from build123d import *

# Parameters (mm, degrees)
SKETCH1_W           = 50
SKETCH1_H           = 80
BOSS_EXTRUDE1_DEPTH = 6
BOSS_EXTRUDE2_DEPTH = 16
FILLET1_R           = 5
FILLET2_R           = 5
SKETCH3_R           = 2.6
CUT_EXTRUDE1_DEPTH  = 10
SKETCH4_W           = 24
SKETCH4_H           = 47.75
CUT_EXTRUDE3_DEPTH  = 20
SKETCH5_W           = 23.965270804
SKETCH5_H           = 10
BOSS_EXTRUDE3_DEPTH = 16
FILLET3_R           = 5


with BuildPart() as part:
    # Sketch1 → Boss-Extrude1 (new body)
    with BuildSketch(Plane(origin=(0, 0, 0), x_dir=(1, 0, 0), z_dir=(0, 1, 0))):
        with Locations((-55.945507312, -78.533333333)):
            Rectangle(SKETCH1_W, SKETCH1_H)
    extrude(amount=BOSS_EXTRUDE1_DEPTH)

    # Sketch2 → Boss-Extrude2 (add)
    with BuildSketch(Plane(origin=(0, 6, 0), x_dir=(1, 0, 0), z_dir=(0, 1, 0))):
        Polygon((-80.945507312, -38.533333333), (-80.945507312, -118.533333333), (-50.945507312, -118.533333333), (-50.945507312, -58.292829883), (-73.945507312, -58.292829883), align=None)
        Polygon((-35.945507312, -44.292829883), (-35.945507312, -118.533333333), (-30.945507312, -118.533333333), (-30.945507312, -38.533333333), (-56.945507312, -44.292829883), align=None)
    extrude(amount=BOSS_EXTRUDE2_DEPTH)

    # Fillet1
    fillet1_edges = [part.edges().sort_by_distance(p)[0] for p in [
        (-50.945507312, 14, 58.292829883),
        (-73.945507312, 14, 58.292829883),
    ]]
    fillet(fillet1_edges, radius=FILLET1_R)

    # Fillet2
    fillet2_edges = [part.edges().sort_by_distance(p)[0] for p in [
        (-35.945507312, 14, 44.292829883),
    ]]
    fillet(fillet2_edges, radius=FILLET2_R)

    # Sketch3 → Cut-Extrude1 (cut)
    with BuildSketch(Plane(origin=(0, 0, 58.292829883), x_dir=(-1, 0, 0), z_dir=(0, 0, -1))):
        with Locations((59.128917582, 16.867919386)):
            Circle(SKETCH3_R)
        with Locations((67.228917582, 16.867919386)):
            Circle(SKETCH3_R)
    extrude(amount=-CUT_EXTRUDE1_DEPTH, mode=Mode.SUBTRACT)

    # Sketch4 → Cut-Extrude3 (cut)
    with BuildSketch(Plane.XZ):
        with Locations((-65.945507312, 92.158333333)):
            Rectangle(SKETCH4_W, SKETCH4_H)
    extrude(amount=-CUT_EXTRUDE3_DEPTH, mode=Mode.SUBTRACT)

    # Sketch5 → Boss-Extrude3 (add)
    with BuildSketch(Plane.XY.offset(68.283333333)):
        with Locations((-65.928142714, 5)):
            Rectangle(SKETCH5_W, SKETCH5_H)
    extrude(amount=BOSS_EXTRUDE3_DEPTH)

    # Fillet3
    fillet3_edges = [part.edges().sort_by_distance(p)[0] for p in [
        (-50.945507312, 14, 118.533333333),
        (-30.945507312, 11, 118.533333333),
        (-80.945507312, 11, 118.533333333),
    ]]
    fillet(fillet3_edges, radius=FILLET3_R)


solid = part.part
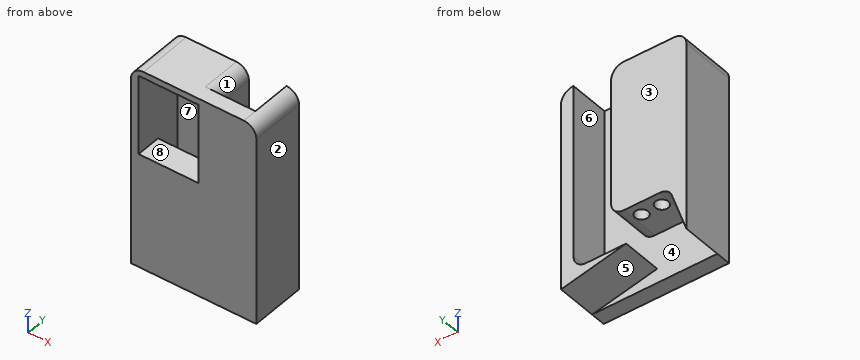
Part model, mm, in its own coordinate system. Face numbers are marked on the shaded views. A direction names the side the tool comes from. Coordinates: 2 decimals unless noted, no trailing zeros. Write each loop counter-clockwise with the first axis right and the second up, starting at its lowest first coordinate (ties: lowest second). Pieces come first, ordered by that corner, then holes. Notation, with made-up numbers: M 58.25,52 L 64.25,52 A24 ccw 64.25,66 Z; hole C 61.25,-34 d5. An arc over 180 degrees is marked long. Return JSON: item names as keys, results as strings.
1. Saw through at A-A, the plane y = 12. Write the cut outline in (x, z), then the cut area to 3 significant figures.
Determined:
{"outline": "M -80.95,38.53 L -75.13,54.96 A5 cw -70.41,58.29 L -55.95,58.29 A5 ccw -50.95,63.29 L -50.95,113.53 A5 ccw -55.95,118.53 L -75.95,118.53 A5 ccw -80.95,113.53 Z; M -56.95,44.29 L -30.95,38.53 L -30.95,113.53 A5 ccw -35.95,118.53 L -35.95,49.29 A5 cw -40.95,44.29 Z; hole M -77.95,68.28 L -53.95,68.28 L -53.95,116.03 L -77.95,116.03 Z", "area": "1,160 mm²"}
2. Flat gauge pins, fed straight in: pin 1 Ø5 at (x, z) = (-45, 89) entering from +Y; pin 2 Ø3 at (x, y) = (-59.5, 11.5) entering from -Z; pin 3 Ø4 at (x, y) = (-59.13, 16.87) entering from -Z. Where does each tip first touch, or does it go through?
Determined:
{"pin 1": "y = 6", "pin 2": "z = 58.29", "pin 3": "z = 116.03"}
3. Probe L1, parallel to Z at x = -68, y = 7; L2, parallel to X at y = 12, z = 69; L3, parallel to Z at x = -61, y = 3. List the from-to ranges inside material, lowest first.
Determined:
{"L1": "58.29 to 84.28, 116.03 to 118.53", "L2": "-80.95 to -77.95, -53.95 to -50.95, -35.95 to -30.95", "L3": "38.53 to 84.28, 116.03 to 118.53"}
4. Saw through at C-C, the plane y = 8. Count the separate pieces of the cut face and the enclosed holes in it, then the cut area to 3 significant figures.
Determined:
{"separate pieces": "2", "enclosed holes": "1", "area": "1,550 mm²"}
5. Saw through at D-D, the plane x = -53. Write the cut outline in (y, z).
Determined:
{"outline": "M 0,38.53 L 6,38.53 L 6,43.42 L 22,43.42 L 22,44.29 L 6,44.29 L 6,59.25 L 22,59.25 L 22,117.57 L 6,117.57 L 6,118.53 L 0,118.53 Z"}
6. Saw through at B-B, the plane z = 106. Write the cut outline in (x, y), then the cut area to 3 significant figures.
Determined:
{"outline": "M -80.95,0 L -77.95,0 L -77.95,20 L -53.95,20 L -53.95,0 L -30.95,0 L -30.95,22 L -35.95,22 L -35.95,6 L -50.95,6 L -50.95,22 L -80.95,22 Z", "area": "380 mm²"}
7. Pull direction X, two halves, no side cores. Call the marked faces 1, 2 and 3: pulls with the +X half, pulls with the -X half, needs draft (parallel to the pull), parting line crosses it, or undercut.
Determined:
{"face 1": "undercut", "face 2": "pulls with the +X half", "face 3": "needs draft"}
8. 3-axis set-ups, long thin cutter, end or side, ignore diameter. For the marked faces 4, 5, 6, 7 and 8: which of +Z, -Z, +X, -X, +Y, -Y reach the whole face in a straight line?
Determined:
{"face 4": "+Y", "face 5": "-Z, +Y", "face 6": "+Z, +Y", "face 7": "none", "face 8": "-Y"}
